The drawing under review shows one solid part. Ordinate dimensions are in mm from its lowest x, y, z. A direction names the side the tool comes from. Coordinates: 2 decimals unless noted, no trailing zeros. Write each loop counter-clockwise with the first axis right and the second up, starting at its lowest first coordinate (ties: lowest second). Pieces come first, ordered by that corner, then holes.
1) Mouldability with a two-part tool opening along X and no side actions: class the marked faces 4, 5 and 6 as released by +X, released by -X, zero draft, split by the parting line, or undercut.
2) Add section B-B, the plane y = 7.25. State the section outline as (x, z) points.
3) For line 1 (X direction, y = 1.75, z = 3.75) (1 decimal); line 2 (X direction, y = 6.25, z = 10.75); line 3 (Z direction, x = 4.25, y = 2.75), list the stretches that pass through material, from the lowest coordinate up.
4) Add section A-A, the plane y = 2.25. State the section outline as (x, z) points (1 decimal).
5) For P1, Ø5, axis at y = 9.5, z = 7.5, coming from the +X side; P2, Ø3, axis at x = 24, z = 3.5, coming from the +Y side; P3, Ø6, axis at y = 8.5, z = 2, coming from the -X side, all flat-tipped, find the tip position at first contact; note any pin that passes through.
6) Add section D-D, the plane x = 16.5. State the section outline as (y, z) points.
7) Add section C-C, the plane z = 1.75. State the section outline as (x, y) points (1 decimal).
8) Machinability: for the marked faces 1, 2 and 3, which of the approach directions +Z, -Z, +X, -X, +Y, -Y give a long, thin tool a straight path to every point of the face, cutting with its end or side? Answer none if there is none.
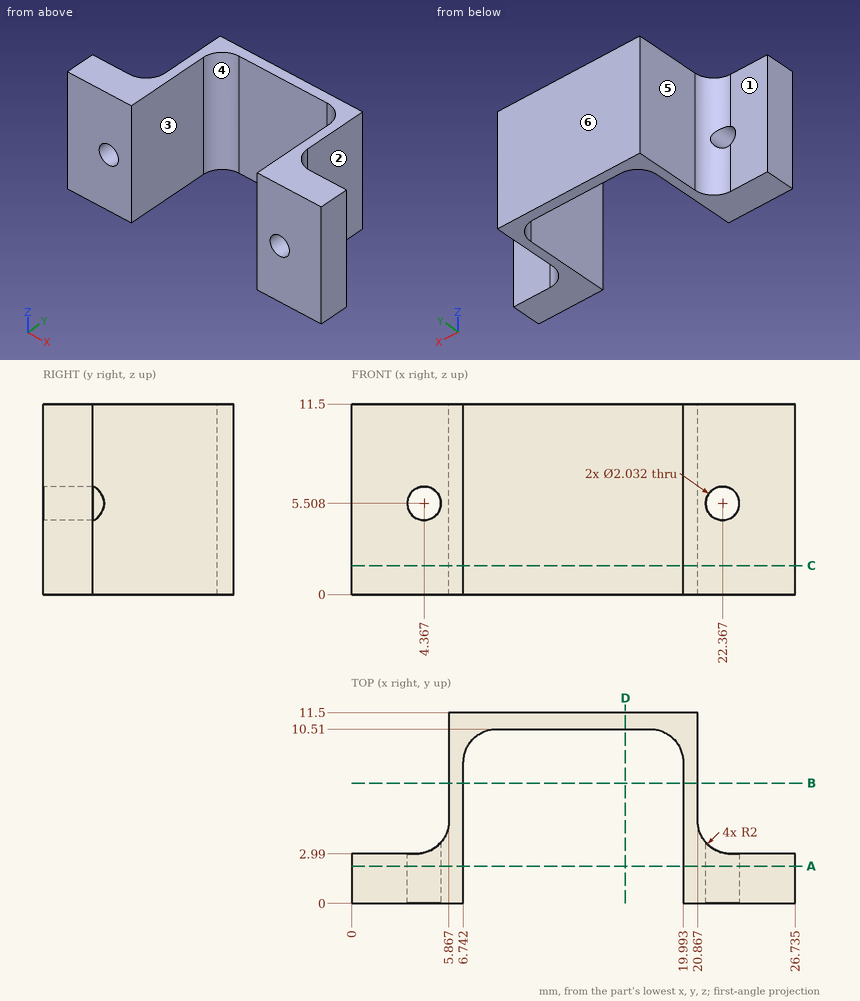
Geometry results:
1. face 4: undercut
1. face 5: released by -X
1. face 6: zero draft
2. outline: (5.87, 0) - (6.74, 0) - (6.74, 11.5) - (5.87, 11.5) - close; (19.99, 0) - (20.87, 0) - (20.87, 11.5) - (19.99, 11.5) - close
3. line 1: x = 0 to 6.7, 20 to 26.7
3. line 2: x = 5.87 to 6.74, 19.99 to 20.87
3. line 3: z = 0 to 4.5, 6.52 to 11.5
4. outline: (0, 0) - (6.7, 0) - (6.7, 11.5) - (0, 11.5) - close; (20, 0) - (26.7, 0) - (26.7, 11.5) - (20, 11.5) - close; hole circle Ø2 at (4.4, 5.5); hole circle Ø2 at (22.4, 5.5)
5. P1: stops at x = 20.87
5. P2: stops at y = 3.02
5. P3: stops at x = 5.87
6. outline: (10.51, 0) - (11.5, 0) - (11.5, 11.5) - (10.51, 11.5) - close
7. outline: (0, 0) - (6.7, 0) - (6.7, 8.5) arc R2 cw to (8.7, 10.5) - (18, 10.5) arc R2 cw to (20, 8.5) - (20, 0) - (26.7, 0) - (26.7, 3) - (22.9, 3) arc R2 cw to (20.9, 5) - (20.9, 11.5) - (5.9, 11.5) - (5.9, 5) arc R2 cw to (3.9, 3) - (0, 3) - close
8. face 1: +Z, -Z, -X, +Y
8. face 2: +Z, -Z, +X, +Y
8. face 3: +Z, -Z, -Y
